Geometry check sheet. Reference: the model listing, model coordinates, mm. Face numbers are marked on the shaded views. Round coordinates to 2 decimals unless told otherwise and drop trailing zeros. Order: outer loops, then holes, each group sorted by start corner. A loop starts at its lowest first (then second) coordinate and runs counter-clockwise, first axis right, second up.
(1) Sectioned sample at B-B (y = -3.75). Record the boundary of the cut face in (x, z).
(2) Sectioned sample at A-A (y = 3). Record the boundary of the cut face in (x, z), plus the area to 3 significant figures.
(3) Release check for a two-part mould opening along Z. For the marked faces 1, 2, 3 and 4 record: +Z half, -Z half, draft (parallel to the pull), parting line (faces both ways), or undercut.
(4) Material ranges on line 1 along X through (y, z) = (4.25, 0.5); line 2 along Y through (x, z) = (45.75, 4); line 3 along X through (y, z) = (-5.75, -2.5), recorded low to high.
(5) Go/stop test with flat-tipped pins: pin 1 (2 mm diameter, centred on y = 0.5, z = -0.5, fed in from -X); pin 2 (2 mm diameter, centred on y = -5, z = -4, fed in from +X); pin 3 (1 mm diameter, centred on x = 45.5, y = -5, fed in from -Z). Record where each tip stops, or that it passes through.
from build123d import *

# Parameters (mm, degrees)
F1_ANGLE = 15


with BuildPart() as f1:
    # F0 (on Top) → F1 (revolve, symmetric)
    with BuildSketch(Plane.XY) as f1_sk:
        with BuildLine():
            Line((40.988395, -3.125822), (47.988395, -9.125822))
            add(Edge.make_bspline(
                [(47.988395, -9.125822), (48.655789, -7.643054), (49.103786, -6.125822)],
                knots=[5.998563, 5.998563, 5.998563, 6.093564, 6.093564, 6.093564], degree=2, weights=[1, 0.998872, 1]))
            Line((49.103786, -6.125822), (42.988395, -1.125822))
            Line((42.988395, -1.125822), (42.988395, 5.874178))
            Line((42.988395, 5.874178), (40.988395, 5.874178))
            Line((40.988395, 5.874178), (40.988395, -3.125822))
        make_face()
    revolve(axis=Axis((0, 4.998505, 0), (0, -1, 0)), revolution_arc=F1_ANGLE / 2)
    revolve(f1_sk.sketch, axis=Axis((0, 4.998505, 0), (0, 1, 0)), revolution_arc=F1_ANGLE / 2)


solid = f1.part
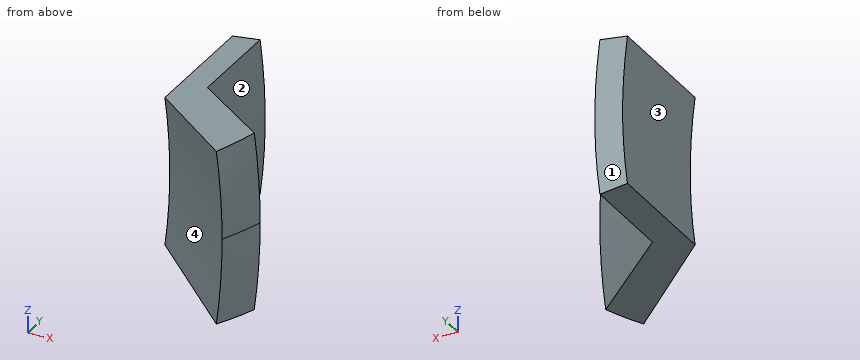
Answer below:
1. outline: (41.36, -5.45) - (45.8, -6.03) arc R46.2 ccw to (45.8, 6.03) - (41.36, 5.45) arc R41.72 cw to start
2. outline: (40.64, -5.35) - (42.62, -5.61) arc R42.99 ccw to (42.62, 5.61) - (40.64, 5.35) arc R40.99 cw to start
2. area: 22.0 mm2
3. face 1: draft
3. face 2: parting line
3. face 3: undercut
3. face 4: undercut
4. line 1: x = 40.99 to 42.99
4. line 2: y = -7.36 to -3.53
4. line 3: x = 43.98 to 48.58
5. pin 1: stops at x = 40.96
5. pin 2: stops at x = 48.79
5. pin 3: stops at z = -6.06
